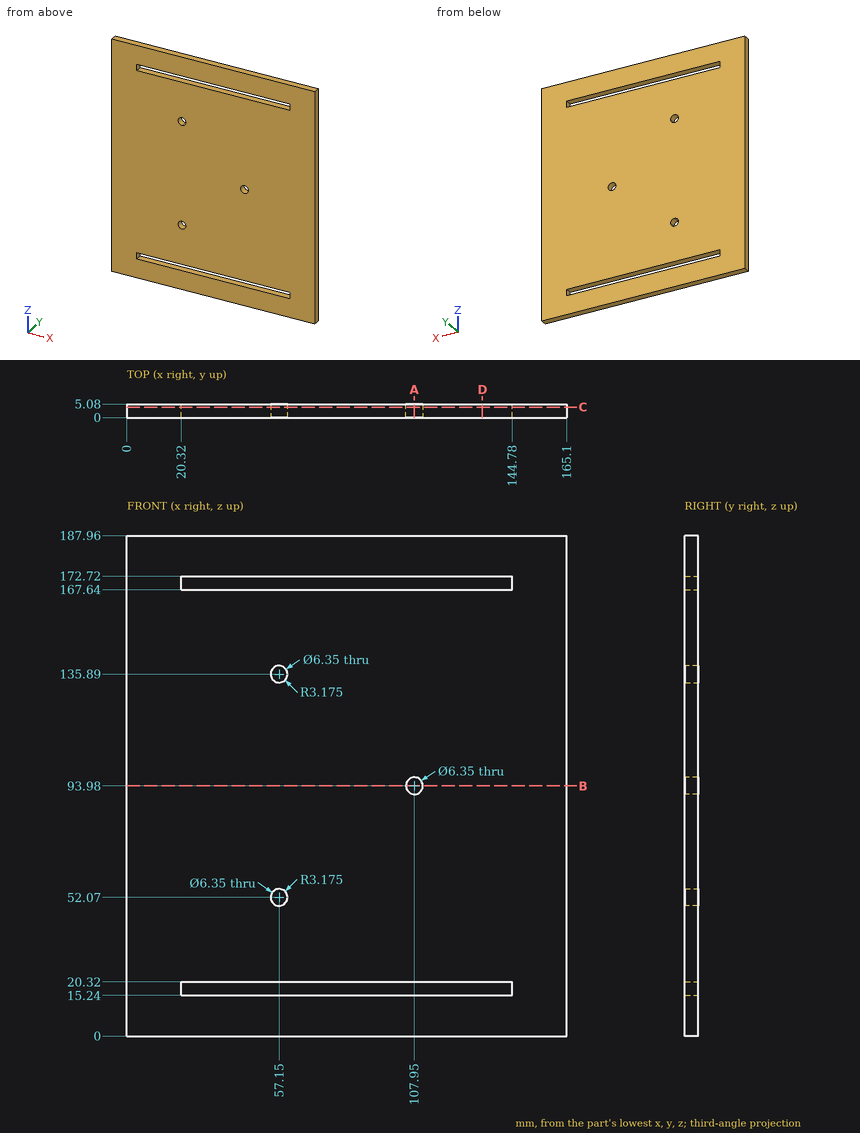
Input: dimensioned drawing with shaded views. Units: mm. Origin: part minimum x, y, z. Round coordinates to 2 decimals unless told otherwise and drop trailing zeros. Order: outer loops, then holes, each group sorted by start corner. A loop starts at its lowest first (then second) coordinate and runs counter-clockwise, first axis right, second up. Notation, with made-up numbers: (35.5, -29) -> (75.5, -29) arc R22 cw to (75.5, -20) -> close; hole circle Ø6 at (60.5, -33). An arc over 180 degrees is marked (long way). Put each result on its own line as item: value. Start each with the question number.
Q1. Line query: probe 1 along Z at (x, y) = (57.15, 3.2) (3 decimals); probe 2 along Z at (x, y) = (66.5, 3.2); probe 3 along Z at (x, y) = (107.95, 2.25) (3 decimals). Output: solid intervals per line, ascending.
Q2. Section D-D on x = 133.5. Return the cut outline in (y, z), and give its area (3 significant figures).
Q3. Section A-A on x = 107.95. Return the cut outline in (y, z) (3 decimals), and give its area (3 significant figures).
Q4. First-contact query: pin 1 (5.5 mm diameter, centred on x = 107.95, z = 93.98, fed in from +Y). Flat tip, straight axial feed; report the tip coordinate or a pass-through.
Q5. Section B-B on z = 93.98. Return the cut outline in (x, y) (3 decimals).
Q6. Section C-C on y = 3.9. Return the cut outline in (x, z) (3 decimals), and give its area (3 significant figures).
Ans:
1. probe 1: z = 0 to 15.24, 20.32 to 48.895, 55.245 to 132.715, 139.065 to 167.64, 172.72 to 187.96
1. probe 2: z = 0 to 15.24, 20.32 to 167.64, 172.72 to 187.96
1. probe 3: z = 0 to 15.24, 20.32 to 90.805, 97.155 to 167.64, 172.72 to 187.96
2. outline: (0, 0) -> (5.08, 0) -> (5.08, 15.24) -> (0, 15.24) -> close; (0, 20.32) -> (5.08, 20.32) -> (5.08, 167.64) -> (0, 167.64) -> close; (0, 172.72) -> (5.08, 172.72) -> (5.08, 187.96) -> (0, 187.96) -> close
2. area: 903 mm2
3. outline: (0, 0) -> (5.08, 0) -> (5.08, 15.24) -> (0, 15.24) -> close; (0, 20.32) -> (5.08, 20.32) -> (5.08, 90.805) -> (0, 90.805) -> close; (0, 97.155) -> (5.08, 97.155) -> (5.08, 167.64) -> (0, 167.64) -> close; (0, 172.72) -> (5.08, 172.72) -> (5.08, 187.96) -> (0, 187.96) -> close
3. area: 871 mm2
4. pin 1: passes through
5. outline: (0, 0) -> (104.775, 0) -> (104.775, 5.08) -> (0, 5.08) -> close; (111.125, 0) -> (165.1, 0) -> (165.1, 5.08) -> (111.125, 5.08) -> close
6. outline: (0, 0) -> (165.1, 0) -> (165.1, 187.96) -> (0, 187.96) -> close; hole (20.32, 15.24) -> (144.78, 15.24) -> (144.78, 20.32) -> (20.32, 20.32) -> close; hole (20.32, 167.64) -> (144.78, 167.64) -> (144.78, 172.72) -> (20.32, 172.72) -> close; hole circle Ø6.35 at (57.15, 52.07); hole circle Ø6.35 at (57.15, 135.89); hole circle Ø6.35 at (107.95, 93.98)
6. area: 29,700 mm2
